from build123d import *

# Parameters (mm, degrees)
DODANIE_WYCI_GNI_CIE3_DEPTH = 11.5
WYTNIJ_WYCI_GNI_CIE1_DEPTH  = 10
DODANIE_WYCI_GNI_CIE4_START = 3
DODANIE_WYCI_GNI_CIE4_DEPTH = 3


with BuildPart() as part:
    # Szkic1 → Dodanie-wyci_gni_cie3 (new body)
    with BuildSketch(Plane.XY):
        with BuildLine():
            Line((20, 2.5), (9.682458366, 2.5))
            ThreePointArc((9.682458366, 2.5), (-10, 0), (9.682458366, -2.5))
            Line((9.682458366, -2.5), (20, -2.5))
            Line((20, -2.5), (20, 2.5))
        make_face()
    extrude(amount=DODANIE_WYCI_GNI_CIE3_DEPTH)

    # Szkic1_6 → Wytnij-wyci_gni_cie1 (cut)
    with BuildSketch(Plane.XY):
        with BuildLine():
            Line((1.55, -2.626785107), (1.55, 2.626785107))
            ThreePointArc((1.55, 2.626785107), (-3.05, 0), (1.55, -2.626785107))
        make_face()
    extrude(amount=WYTNIJ_WYCI_GNI_CIE1_DEPTH, mode=Mode.SUBTRACT)

    # Szkic2 → Dodanie-wyci_gni_cie4 (add)
    with BuildSketch(Plane(origin=(0, 0, 0), x_dir=(-1, 0, 0), z_dir=(0, 0, -1)).offset(DODANIE_WYCI_GNI_CIE4_START)):
        with BuildLine():
            ThreePointArc((-9.682458366, -2.5), (1.260042925, -9.920296963), (10, 0))
            ThreePointArc((10, 0), (1.260042925, 9.920296963), (-9.682458366, 2.5))
            ThreePointArc((-9.682458366, 2.5), (-10, 0), (-9.682458366, -2.5))
        make_face()
        with BuildLine():
            ThreePointArc((-1.55, -2.626785107), (-3.05, 0), (-1.55, 2.626785107))
            ThreePointArc((-1.55, 2.626785107), (1.512448346, 2.648584528), (3.05, 0))
            ThreePointArc((3.05, 0), (1.512448346, -2.648584528), (-1.55, -2.626785107))
        make_face(mode=Mode.SUBTRACT)
    extrude(amount=-DODANIE_WYCI_GNI_CIE4_DEPTH)


solid = part.part
Geometry: final body of the model. Coordinates: model frame, mm. A direction names the side the tool comes from. Round coordinates to 2 decimals unless told otherwise and drop trailing zeros. Loops run counter-clockwise (first coordinate to the right, second up) from the corner with the lowest first, then second, coordinate; pieces in that order, holes last. Notation, with made-up numbers: (-38.5, 21.5) -> (6.5, 21.5) arc R16 cw to (6.5, 25.5) -> close; hole circle Ø4 at (-3.75, 18). An arc over 180 degrees is marked (long way). One line per question, with ' | ' between items. Start each with the question number.
1. Section C-C on y = -1. Output: boundary loops of the cut face in (x, z), and give its area (3 significant figures).
2. Set-up query: faces 1 (the face through (1.55, 0, 5)), 2 (the face through (1, 0, 11.5)), 3 (the face through (15, 2.5, 6)), 4 (the face through (15, -2.5, 6)). Return all of +Z, -Z, +X, -X, +Y, -Y with unobstructed straight access to the full face (end or side cutting, diameter ignored); none if empty.
3. Mould query, pull axis X, two halves, no side actions, for faces 5 (the face through (20, 0, 6)), 6 (the face through (2, 0, 0)), 7 (the face through (2.4, 2.4, -3)). Classes: pulls with the +X half, pulls with the -X half, needs draft (parallel to the pull), parting line crosses it, or undercut.
4. Section D-D on z = 3.5. Output: boundary loops of the cut face in (x, y).
5. Contact query for flat-ended pins moving along their axis: pin 1 (1.5 mm diameter, centred on x = 14, y = -1, fed in from -Z); pin 2 (8.5 mm diameter, centred on x = 17, z = 3, fed in from -Y); pin 3 (2 mm diameter, centred on y = -8, z = 2, fed in from -X). Output: stop coordinate, or through.
6. Section A-A on z = -1.75. Output: boundary loops of the cut face in (x, y).
7. Line query: line 1 along X through (y, z) = (0, 5.25); line 2 along Y through (x, z) = (0, 6). Output: solid intervals per line, ascending. Write a range as [from, to].
8. Section B-B on x = 0. Output: boundary loops of the cut face in (y, z), and give its area (3 significant figures).
Returned:
1) outline: (-9.95, -3) -> (-2.88, -3) -> (-2.88, 10) -> (1.55, 10) -> (1.55, 0) -> (2.88, 0) -> (2.88, -3) -> (9.95, -3) -> (9.95, 0) -> (20, 0) -> (20, 11.5) -> (-9.95, 11.5) -> close | area: 343 mm2
2) face 1: -Z | face 2: +Z, +X, -X, +Y, -Y | face 3: +Z, -Z, +X, +Y | face 4: +Z, -Z, +X, -Y
3) face 5: pulls with the +X half | face 6: undercut | face 7: needs draft
4) outline: (9.68, -2.5) -> (20, -2.5) -> (20, 2.5) -> (9.68, 2.5) arc R10 ccw (long way) to start; hole (1.55, -2.63) -> (1.55, 2.63) arc R3.05 ccw (long way) to start
5) pin 1: stops at z = 0 | pin 2: stops at y = -2.5 | pin 3: stops at x = -7.14
6) outline: circle Ø20 at (0, 0); hole circle Ø6.1 at (0, 0)
7) line 1: x = [-10, -3.05], [1.55, 20] | line 2: y = [-10, -3.05], [3.05, 10]
8) outline: (-10, -3) -> (-3.05, -3) -> (-3.05, 10) -> (3.05, 10) -> (3.05, -3) -> (10, -3) -> (10, 11.5) -> (-10, 11.5) -> close | area: 211 mm2
